Could you check a few things on this model? Use its own coordinates, in mm. A direction names the side the tool comes from. Give positions to 0.01 mm unless a question says otherwise; leave off trailing zeros. Loops run counter-clockwise (first coordinate to the right, second up) from the corner with the lowest first, then second, coordinate; pieces in that order, holes last. Notation, with made-up numbers: (43, 69) - (87, 69) arc R16 ccw to (87, 84) - close; hole circle Ø3 at (-29.5, -11.5). An arc over 180 degrees is marked (long way). Write each question's results on one line, items separated by ' | '. Start each with the question number.
1) I'm going to push flat-ended pins straight in: pin 1 (2.5 mm diameter, centred on x = 6.5, z = 5.5, fed in from -Y); pin 2 (1 mm diameter, centred on x = 4, y = 13, fed in from +Z). Where does each tip first touch, or does it pass through?
2) I want a section at D-D, the plane x = -9.5. Write out the boundary of the cut face in (y, z), and give its area (3 significant figures).
3) If I drill on probe 1 along X at (y, z) = (37, 4); probe 2 along Z at (x, y) = (9.25, 17.5); probe 3 along Y at (x, z) = (-0.5, 3), over which ranges is the centre line in solid material (lowest first)? Write a range as [from, to].
4) I want a section at C-C, the plane z = 2.75. Write out the boundary of the cut face in (x, y).
5) On a 3-axis mill with a long thin cutter (end or side, diameter ignored), from which of +Z, -Z, +X, -X, +Y, -Y can I reach the whole of each face in a straight line? I mean faces 1 (the face through (-3, 15, 3.75)), 2 (the face through (1.5, 23, 3)), 3 (the face through (-7, 33, 6.8)). Say none if no direction works.
6) I want a section at B-B, the plane z = 4.5. Write out the boundary of the cut face in (x, y).
7) I want a section at A-A, the plane y = 14. Write out the boundary of the cut face in (x, z), and give its area (4 significant figures).
8) If we mould it in two halves opening along X, with no side actions, what happens to faces 4 (the face through (-13, 20, 2)), 5 (the face through (7, 30, 5)), 6 (the face through (0, 5, 2)), 7 (the face through (-1.5, 22, 3))? For each: +X half, -X half, draft (parallel to the pull), parting line (faces both ways), or undercut.
from build123d import *

# Parameters (mm, degrees)
F0_W     = 11.5
F0_H     = 25
F0_W_2   = 1.5
F0_H_2   = 5
F1_DEPTH = 3.75
F0_H_3   = 10
F2_DEPTH = 6.8
F3_SIZE  = 5


with BuildPart() as f1:
    # F0 (on Top) → F1 (new body)
    with BuildSketch(Plane.XY):
        with Locations((-7.25, 17.5)):
            Rectangle(F0_W, F0_H)
        Polygon((1.5, 30), (1.5, 5), (13, 4.9315184347), (13, 30), align=None)
        Polygon((1.5, 5), (1.5, 0), (13, 0), (13, 4.9315184347), align=None)
        with Locations((0.75, 2.5)):
            Rectangle(F0_W_2, F0_H_2)
        with Locations((-0.75, 2.5)):
            Rectangle(F0_W_2, F0_H_2)
        with Locations((-7.25, 2.5)):
            Rectangle(F0_W, F0_H_2)
    extrude(amount=F1_DEPTH)

    # F0 (on Top) → F2 (join)
    with BuildSketch(Plane.XY):
        with Locations((-7.25, 35)):
            Rectangle(F0_W, F0_H_3)
        with Locations((7.25, 35)):
            Rectangle(F0_W, F0_H_3)
    extrude(amount=F2_DEPTH)

    # F3
    f3_edges = [f1.edges().sort_by_distance(p)[0] for p in [
        (-7.25, 40, 6.8),
        (7.25, 40, 6.8),
    ]]
    chamfer(f3_edges, length=F3_SIZE)


solid = f1.part
Answers:
1) pin 1: stops at y = 30 | pin 2: stops at z = 3.75
2) outline: (0, 0) - (40, 0) - (40, 1.8) - (35, 6.8) - (30, 6.8) - (30, 3.75) - (0, 3.75) - close | area: 168 mm2
3) probe 1: x = [-13, -1.5], [1.5, 13] | probe 2: z = [0, 3.75] | probe 3: y = [0, 5]
4) outline: (-13, 0) - (13, 0) - (13, 39.05) - (1.5, 39.05) - (1.5, 5) - (-1.5, 5) - (-1.5, 39.05) - (-13, 39.05) - close
5) face 1: +Z, +X, -X, -Y | face 2: +Z, -Z, +Y | face 3: +Z, +X, -X, +Y, -Y
6) outline: (-13, 30) - (-1.5, 30) - (-1.5, 37.3) - (-13, 37.3) - close; (1.5, 30) - (13, 30) - (13, 37.3) - (1.5, 37.3) - close
7) outline: (-13, 0) - (-1.5, 0) - (-1.5, 3.75) - (-13, 3.75) - close; (1.5, 0) - (13, 0) - (13, 3.75) - (1.5, 3.75) - close | area: 86.25 mm2
8) face 4: -X half | face 5: draft | face 6: undercut | face 7: undercut
